from build123d import *

# Parameters (mm, degrees)
SKETCH1_W               = 127
SKETCH1_H               = 127
BOSS_EXTRUDE1_DEPTH     = 12.7
CUT_EXTRUDE1_DEPTH      = 137.061310783
CUT_EXTRUDE1_DEPTH_BACK = 137.061310783
SKETCH3_W               = 76.2
SKETCH3_H               = 76.2
CUT_EXTRUDE2_DEPTH      = 137.061310783
CUT_EXTRUDE2_DEPTH_BACK = 137.061310783
SKETCH4_R               = 6.35


with BuildPart() as part:
    # Sketch1 → Boss-Extrude1 (new body)
    with BuildSketch(Plane.XY):
        with Locations((28.396629213, 36.030898876)):
            Rectangle(SKETCH1_W, SKETCH1_H)
    extrude(amount=-BOSS_EXTRUDE1_DEPTH)

    # Sketch3 → Cut-Extrude1 (cut, two sides: drawn at the far end of the back side and taken through both)
    with BuildSketch(Plane.XY.offset(-CUT_EXTRUDE1_DEPTH_BACK)):
        with Locations((2.996629213, 10.630898876)):
            Rectangle(SKETCH3_W, SKETCH3_H)
    extrude(amount=CUT_EXTRUDE1_DEPTH + CUT_EXTRUDE1_DEPTH_BACK, mode=Mode.SUBTRACT)

    # Sketch4 → Cut-Extrude2 (cut, two sides: drawn at the far end of the back side and taken through both)
    with BuildSketch(Plane.XY.offset(-CUT_EXTRUDE2_DEPTH_BACK)):
        with Locations((72.846629213, 80.480898876)):
            Circle(SKETCH4_R)
    extrude(amount=CUT_EXTRUDE2_DEPTH + CUT_EXTRUDE2_DEPTH_BACK, mode=Mode.SUBTRACT)


solid = part.part
Input: part model. Units: mm. Frame: model coordinates. A direction names the side the tool comes from. Give positions to 0.01 mm unless a question says otherwise; leave off trailing zeros. Loops run counter-clockwise (first coordinate to the right, second up) from the corner with the lowest first, then second, coordinate; pieces in that order, holes last. Notation, with made-up numbers: M -4,87 L 15,87 A29 ccw 15,109 Z; hole C -14.5,-4 d6. An arc over 180 degrees is marked long. Use one line per item in the form item = value.
1. First-contact query: pin 1 (14.5 mm diameter, centred on x = 72.85, y = 80.48, fed in from -Z); pin 2 (3 mm diameter, centred on x = 27, z = -2, fed in from -Y); pin 3 (4 mm diameter, centred on y = 29, z = -7.5, fed in from -X). Flat tips, straight axial feed; report the tip coordinate or a pass-through.
Numbers:
pin_1 = -12.7
pin_2 = 48.73
pin_3 = 41.1
2. Reachability of faces 1 (the face through (42, 51, 0)), 2 (the face through (2, 48.731, -6)) from +Z, -Z, +X, -X, +Y, -Y: full face, straight path, thin tool, end or side. Return the list, or none.
Numbers:
face_1 = +Z, +X, -X, +Y, -Y
face_2 = +Z, -Z, -X, -Y
3. Section query B-B, the plane z = -8.25. Return the cut outline in (x, y), and give its area (3 significant figures).
Numbers:
outline = M -35.1,48.73 L 41.1,48.73 L 41.1,-27.47 L 91.9,-27.47 L 91.9,99.53 L -35.1,99.53 Z; hole C 72.85,80.48 d12.7
area = 10,200 mm²
4. Section query C-C, the plane y = 31. Return the cut outline in (x, z), and give its area (3 significant figures).
Numbers:
outline = M 41.1,-12.7 L 91.9,-12.7 L 91.9,0 L 41.1,0 Z
area = 645 mm²
5. Line query: L1, parallel to Y at x = -26.5, z = -2.5; L2, parallel to X at y = 46.5, z = -0.75; L3, parallel to X at y = 82.5, z = -2. Output: solid intervals per line, ascending.
Numbers:
L1 = 48.73 to 99.53
L2 = 41.1 to 91.9
L3 = -35.1 to 66.83, 78.87 to 91.9
6. Section query D-D, the plane x = -11.5. Return the cut outline in (y, z).
Numbers:
outline = M 48.73,-12.7 L 99.53,-12.7 L 99.53,0 L 48.73,0 Z
7. Section query A-A, the plane y = 82.5. Return the cut outline in (x, z), and give its area (3 significant figures).
Numbers:
outline = M -35.1,-12.7 L 66.83,-12.7 L 66.83,0 L -35.1,0 Z; M 78.87,-12.7 L 91.9,-12.7 L 91.9,0 L 78.87,0 Z
area = 1,460 mm²
8. Pull-direction query (X, two-part tool) for faces 3 (the face through (41.097, 10, -6)), 4 (the face through (66.503, 80.76, -6.439)), 5 (the face through (28, 99.531, -6)); classes: released by +X, released by -X, zero draft, split by the parting line, or undercut.
Numbers:
face_3 = released by -X
face_4 = undercut
face_5 = zero draft
